Input: part model. Units: mm. Frame: model coordinates. Give positions to 0.01 mm unless a question says otherwise; leave off trailing zeros. Loops run counter-clockwise (first coordinate to the right, second up) from the corner with the lowest first, then second, coordinate; pieces in that order, holes last. Notation, with made-up numbers: M -35.5,20 L 4.5,20 A31 ccw 4.5,53 Z; hole C -5,43 d2. An arc over 180 degrees is marked long. Use CSV: the item, a comma, the result in double quotes. Start each with the question number.
Q1. Section B-B, the plane y = 35.5. Output: boundary loops of the cut face in (x, z).
Q2. Material intervals for line 1 along X through (y, z) = (95, -46); line 2 along X through (y, z) = (80, -1); line 3 along Y through (x, z) = (-389, 5) (3 decimals), sorted ascending.
Q3. Pin query (flat end, axial travel): pin 1 (5 mm diameter, centred on y = 47, z = -11.5, fed in from -X). Return the tip coordinate at first contact, or that it passes through.
Q4. Section A-A, the plane z = -32.5. Output: boundary loops of the cut face in (x, y), plus the area to 3 significant figures.
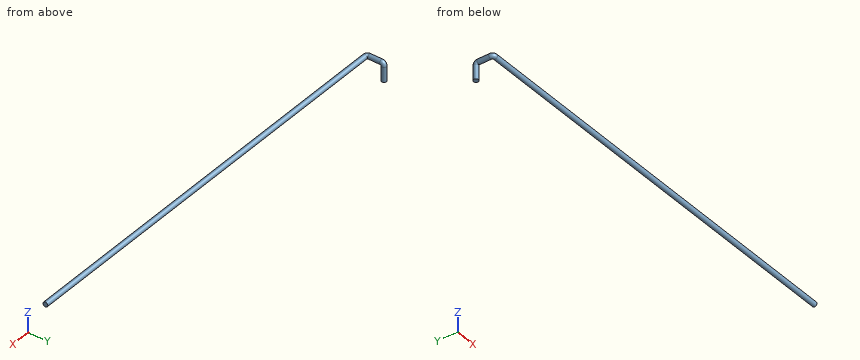
from build123d import *

# Parameters (mm, degrees)
CROQUIS1_R = 13.7


with BuildPart() as part:
    # Barrer1: sweep along a curve in space
    with BuildLine() as barrer1_path:
        Line((0, 0, 0), (-2374, 0, 0))
        ThreePointArc((-2374, 0, 0), (-2384.606601718, 4.393398282, 0), (-2389, 15, 0))
        Line((-2389, 15, 0), (-2389, 83, 0))
        ThreePointArc((-2389, 83, 0), (-2389, 93.606601718, -4.393398282), (-2389, 98, -15))
        Line((-2389, 98, -15), (-2389, 98, -100))
    # Croquis1 → Barrer1 (sweep)
    with BuildSketch(Plane(origin=(0, 0, 0), x_dir=(0, 0, -1), z_dir=(1, 0, 0))):
        Circle(CROQUIS1_R)
    sweep(path=barrer1_path.line)


solid = part.part
A:
1,outline,"C -2389,0 d27.4"
2,line 1,"-2402.37 to -2375.63"
2,line 2,"-2402.66 to -2375.34"
2,line 3,"-12.755 to 12.755"
3,pin 1,"x = -2399.33"
4,outline,"C -2389,98 d27.4"
4,area,"590 mm^2"
